Answer from the drawing. Dimensions are ordinates in mm from the lowest x, y and z of the part. A direction names the side the tool comes from. Round coordinates to 2 decimals unless told otherwise and drop trailing zeros. Write each loop counter-clockwise with the first axis right and the second up, starting at its lowest first coordinate (ties: lowest second). Pieces come first, ordered by that corner, then holes. Notation, with made-up numbers: (18.5, 60.5) - (56.5, 60.5) arc R23 ccw to (56.5, 89.5) - close; hole circle Ø4 at (-18.5, -22.5). An arc over 180 degrees is marked (long way). Answer in a Markdown table with one row per item.
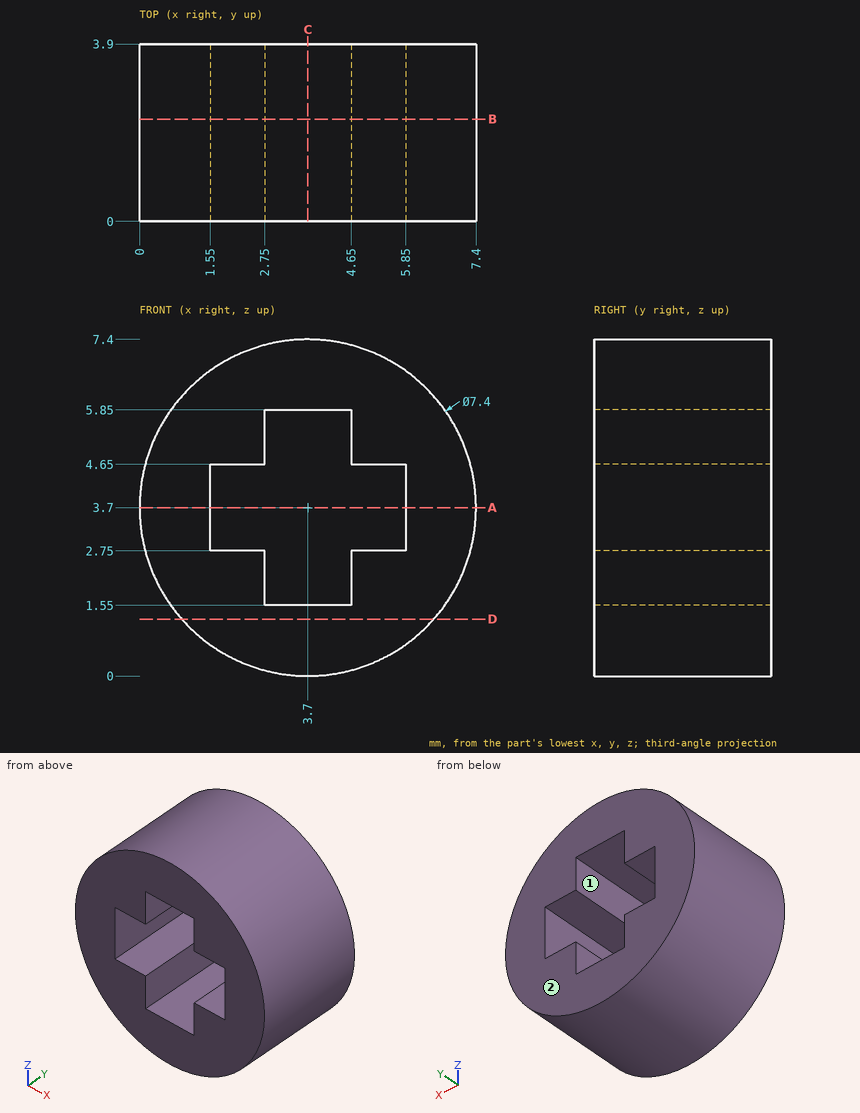
(1) Section B-B (y = 2.25) is taken. Give the vertices of the cut face in (x, z).
Checked values:
| item | result |
|---|---|
| outline | circle Ø7.4 at (3.7, 3.7); hole (1.55, 2.75) - (2.75, 2.75) - (2.75, 1.55) - (4.65, 1.55) - (4.65, 2.75) - (5.85, 2.75) - (5.85, 4.65) - (4.65, 4.65) - (4.65, 5.85) - (2.75, 5.85) - (2.75, 4.65) - (1.55, 4.65) - close |
(2) Section A-A (z = 3.7) is taken. Give the vertices of the cut face in (x, y), and give its area (3 significant figures).
Checked values:
| item | result |
|---|---|
| outline | (0, 0) - (1.55, 0) - (1.55, 3.9) - (0, 3.9) - close; (5.85, 0) - (7.4, 0) - (7.4, 3.9) - (5.85, 3.9) - close |
| area | 12.1 mm2 |
(3) Section C-C (x = 3.7) is taken. Give the vertices of the cut face in (y, z), and give its area (3 significant figures).
Checked values:
| item | result |
|---|---|
| outline | (0, 0) - (3.9, 0) - (3.9, 1.55) - (0, 1.55) - close; (0, 5.85) - (3.9, 5.85) - (3.9, 7.4) - (0, 7.4) - close |
| area | 12.1 mm2 |
(4) Find the intervals of material crossed by line 1 (Z direction, x = 3.75, y = 1.4); line 2 (Z direction, x = 5.75, y = 1.3), in increasing order.
Checked values:
| item | result |
|---|---|
| line 1 | z = 0 to 1.55, 5.85 to 7.4 |
| line 2 | z = 0.62 to 2.75, 4.65 to 6.78 |
(5) Section D-D (z = 1.25) is taken. Give the vertices of the cut face in (x, y).
Checked values:
| item | result |
|---|---|
| outline | (0.93, 0) - (6.47, 0) - (6.47, 3.9) - (0.93, 3.9) - close |
(6) Flat-ended cylindrical pins translate along their axes: pin 1 (1.3 mm diameter, centred on y = 1.5, z = 5, fed in from -X); pin 2 (1.3 mm diameter, centred on y = 1.5, z = 2, fed in from -X); pin 3 (1.3 mm diameter, centred on x = 5, y = 2.5, fed in from -Z). Find the tip coordinate at first contact, or state that the pin passes through.
Checked values:
| item | result |
|---|---|
| pin 1 | stops at x = 0.06 |
| pin 2 | stops at x = 0.15 |
| pin 3 | stops at z = 0.06 |
(7) For the marked faces 1 and 2, determine the directions among +Z, -Z, +X, -X, +Y, -Y from which every point of the face is accessible in a straight line to the end or side of a thin tool.
Checked values:
| item | result |
|---|---|
| face 1 | +Y, -Y |
| face 2 | +Z, -Z, +X, -X, +Y |
